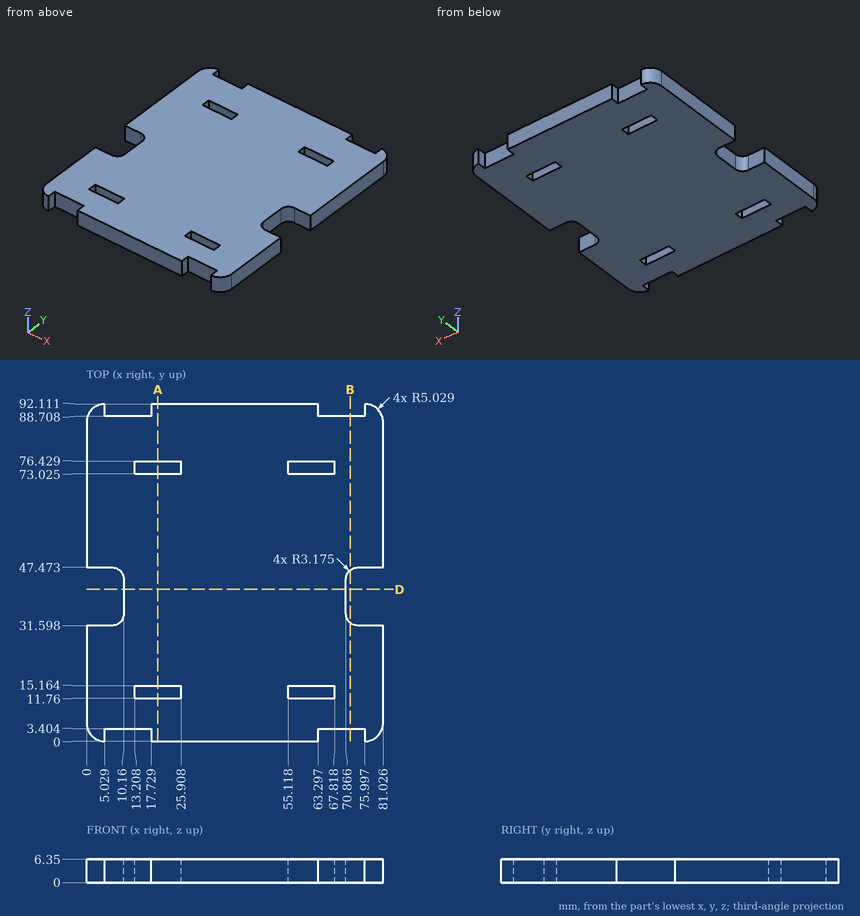
Print and shaded views of the part. All mm, measured from the part's lowest x, y and z. Round coordinates to 2 decimals unless told otherwise and drop trailing zeros. Write each loop counter-clockwise with the first axis right and the second up, starting at its lowest first coordinate (ties: lowest second). Pieces come first, ordered by that corner, then holes. Notation, with made-up numbers: (59, -30.5) - (71, -30.5) arc R20 cw to (71, -12.5) - close; hole circle Ø2 at (-18, -3.75). An arc over 180 degrees is marked (long way). One line per question, with ' | ' between items.
1. Drop flat-ended pins along their axis: pin 1 Ø3 at (x, z) = (71, 4.5) entering from +Y; pin 2 Ø3 at (x, z) = (64, 3) entering from +Y; pin 3 Ø1.7 at (y, z) = (89.5, 4) entering from +X (1 decimal); pin 4 Ø1 at (y, z) = (1.5, 1.5) entering from -X (1 decimal). Give the stop position or say it passes through.
Results are:
pin 1: y = 88.71 | pin 2: y = 92.11 | pin 3: x = 80.8 | pin 4: x = 1
2. Band-saw the part on A-A, the plane x = 19.5. Give the number of separate pieces and of enclosed holes in the cut face.
Results are:
separate pieces: 3 | enclosed holes: 0
3. Band-saw the part on B-B, the plane x = 72. Write the cut outline in (y, z).
Results are:
outline: (3.4, 0) - (32.34, 0) - (32.34, 6.35) - (3.4, 6.35) - close; (46.73, 0) - (88.71, 0) - (88.71, 6.35) - (46.73, 6.35) - close
4. Band-saw the part on D-D, the plane y = 41.5. Write the cut outline in (x, z).
Results are:
outline: (10.16, 0) - (70.87, 0) - (70.87, 6.35) - (10.16, 6.35) - close
5. Drill centre lines: line 1 along X through (y, z) = (13.5, 3.5); line 2 along Y through (x, z) = (16, 3.5) (1 decimal); line 3 along Y through (x, z) = (59, 1.5) (1 decimal). Where is each one in solid material? Low to high. Write a range as from..to.
Results are:
line 1: 0..13.21, 25.91..55.12, 67.82..81.03 | line 2: 3.4..11.8, 15.2..73, 76.4..88.7 | line 3: 0..11.8, 15.2..73, 76.4..92.1
